```python
from build123d import *

# Parameters (mm, degrees)
SKETCH3_R          = 3
BODY_DEPTH         = 57
CUT_KEY_DEPTH      = 58.15767665
CUT_KEY_DEPTH_BACK = 58.15767665
SKETCH7_W          = 2.875
SKETCH7_H          = 2.875


with BuildPart() as part:
    # Sketch3 → body (new body)
    with BuildSketch(Plane.XY):
        Circle(SKETCH3_R)
    extrude(amount=-BODY_DEPTH)

    # Sketch5 → cut-thread (revolve, cut)
    with BuildSketch(Plane(origin=(0, 0, 0), x_dir=(0, 0, -1), z_dir=(1, 0, 0)), mode=Mode.PRIVATE) as cut_thread_sk:
        Polygon((15.625, 2.350480947), (16, 3), (16, 5.821231691), (0, 5.821231691), (0, 3), (15.25, 3), align=None)
    revolve(cut_thread_sk.sketch.rotate(Axis((0, 0, 0), (0, 0, -1)), 90), axis=Axis((0, 0, 0), (0, 0, -1)), mode=Mode.SUBTRACT)

    # Sketch7 → cut-key (cut, two sides: drawn at the far end of the back side and taken through both)
    with BuildSketch(Plane(origin=(0, 0, 0), x_dir=(1, 0, 0), z_dir=(0, 1, 0)).offset(-CUT_KEY_DEPTH_BACK)):
        with Locations((3.9375, 17.0625)):
            Rectangle(SKETCH7_W, SKETCH7_H)
        with Locations((-3.9375, 17.0625)):
            Rectangle(SKETCH7_W, SKETCH7_H)
    extrude(amount=CUT_KEY_DEPTH + CUT_KEY_DEPTH_BACK, mode=Mode.SUBTRACT)


solid = part.part
```
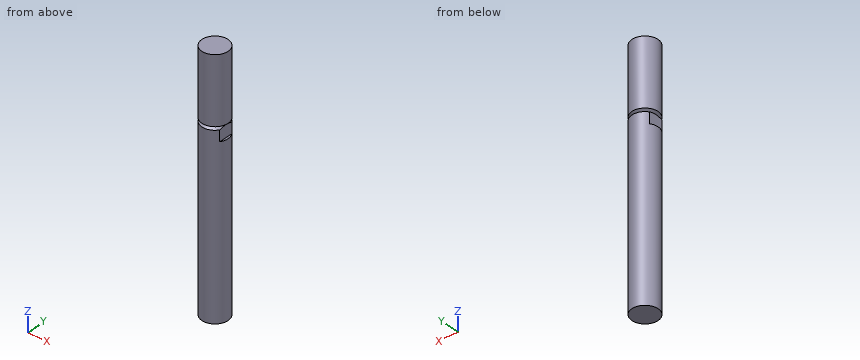
Source: CAD feature listing. Evaluate the final solid. Frame: model axes, mm. Round coordinates to 2 decimals unless told otherwise and drop trailing zeros. Loops run counter-clockwise (first coordinate to the right, second up) from the corner with the lowest first, then second, coordinate; pieces in that order, holes last.
(1) Section query A-A (z = -45). Output: boundary loops of the cut face in (x, y).
From the geometry:
outline: circle Ø6 at (0, 0)
(2) Contact query for flat-ended pins moving along their axis: pin 1 Ø1 at (x, z) = (2, -6.5) entering from -Y; pin 2 Ø1 at (y, z) = (-2, -40) entering from -X; pin 3 Ø1.5 at (x, z) = (1, -17.5) entering from +Y. Output: stop coordinate, or through.
From the geometry:
pin 1: stops at y = -2.6
pin 2: stops at x = -2.6
pin 3: stops at y = 2.99
(3) Material intervals for probe 1 along X at (y, z) = (-1.65, -2.5); probe 2 along Y at (x, z) = (0.25, -14.5); probe 3 along Z at (x, y) = (0.35, 2.7), sorted ascending.
From the geometry:
probe 1: x = -2.51 to 2.51
probe 2: y = -2.99 to 2.99
probe 3: z = -57 to -15.84, -15.41 to 0
